Could you check a few things on this model? Use its own coordinates, in mm. A direction names the side the tool comes from. Give positions to 0.01 mm unless a question says otherwise; leave off trailing zeros. Loops run counter-clockwise (first coordinate to the right, second up) from the corner with the lowest first, then second, coordinate; pieces in that order, holes last. Notation, with made-up numbers: (44, -33.5) - (66, -33.5) arc R37 ccw to (66, 4.5) - close; hole circle Ø2 at (30, 29). An arc over 180 degrees is marked (long way). Write each question's results on one line, items separated by ' | '. Start each with the question number.
(1) Suppose I cut it at C-C (z = -11). Please give me the cut outline in (x, y).
(2) Suppose I cut it at A-A (z = -4.75). Please give me the cut outline in (x, y).
(3) If we mould it in two halves opening along Y, with no side actions, what happens to faces 6 (the face through (-6, 0, -6)), 7 (the face through (-7.3, 6, -10.3)), 8 (the face through (-1.25, 5, -6))? For each: released by +Y, released by -Y, zero draft, split by the parting line, or undercut.
(4) For pin 1 (1.2 mm diameter, centred on x = -6, y = 5, fed in from -Z); pin 2 (1.6 mm diameter, centred on x = -6, y = 5, fed in from +Z); pin 3 (0.8 mm diameter, centred on y = 5, z = -8.5, fed in from +X), each with a flat end and sliding along its axis, tell me the tip position at first contact or that it passes through.
(5) Suppose I cut it at B-B (x = -8.25). Please give me the cut outline in (y, z), and give its area (4 significant figures).
(6) On a 3-axis mill with a long thin cutter (end or side, diameter ignored), from which of +Z, -Z, +X, -X, +Y, -Y can I reach the whole of each face in a straight line? I mean faces 1 (the face through (0, 2, -6)), 2 (the face through (-6, 2, -12.55)), 3 (the face through (-6, 5, -11.25)), 4 (the face through (-6, 5, -1.25)), 5 (the face through (-11.25, 5, -6)). Say none if no direction works.
(7) Suppose I cut it at D-D (x = -0.75). Please give me the cut outline in (y, z), and give its area (3 significant figures).
(8) I need wall thicknesses on line 1 (Y direction, x = -8.75, z = -0.75); line 2 (Z direction, x = -1.75, y = 4.4). Which ranges of each line are inside material? Lowest first, please.
Autodesk Inventor part; units mm, degrees
ref_plane "YZ Plane" through (0, 0, 0) normal (1, 0, 0) x (0, 1, 0)
ref_plane "XZ Plane" through (0, 0, 0) normal (0, 1, 0) x (-1, 0, 0)
ref_plane "XY Plane" through (0, 0, 0) normal (0, 0, 1) x (1, 0, 0)
sketch "Sketch1" plane through (0, 0, 0) normal (0, 1, 0) x (-1, 0, 0)
  line L0 (0, 0) -> (12.5, 0)
  line L1 (12.5, 0) -> (12.5, -12.55)
  line L2 (12.5, -12.55) -> (0, -12.55)
  line L3 (0, -12.55) -> (0, 0)
  dimension "d0" = 12.5
  dimension "d1" = 12.55
extrude "Extrusion1" add sketch "Sketch1" along normal blind 4
sketch "Sketch2" plane through (0, 4, 0) normal (0, 1, 0) x (1, 0, 0)
  line L0 (-11.25, 1.25) -> (-1.25, 1.25)
  line L1 (-1.25, 1.25) -> (-1.25, 11.25)
  line L2 (-1.25, 11.25) -> (-11.25, 11.25)
  line L3 (-11.25, 11.25) -> (-11.25, 1.25)
  line L4 (-12.5, 0) -> (0, 0)
  line L5 (-12.5, 12.55) -> (-12.5, 0)
  dimension "d4" = 10
  dimension "d5" = 10
  dimension "d6" = 1.25
  dimension "d7" = 1.25
extrude "Extrusion2" add sketch "Sketch2" along normal blind 2
ref_plane "Work Plane1" through (-11.25, 4, -6.25) normal (0, 0, 1) x (1, 0, 0)
sketch "Sketch3" plane through (-11.25, 4, -6.25) normal (0, 0, 1) x (1, 0, 0)
  line L0 (10, 0) -> (0, 0)
  line L1 (10, 0) -> (10, 2)
  line L2 (0, 2) -> (10, 2)
  line L3 (0, 0) -> (0, 2)
  line L4 (5, 2) -> (5, 1.5)
  line L5 (5, 2) -> (9, 2)
  line L6 (5, 2) -> (1, 2)
  arc A0 (1, 2) -> (9, 2) centre (5, 17.75) ccw
  point P0 (11.25, -4)
  dimension "d10" = 0.5
  dimension "d11" = 4
  dimension "d12" = 4
revolve "Revolution1" cut sketch "Sketch3" angle 360 about axis through (-6.25, 6, -6.25) along (0, -1, 0) picked at (7.2273, 1.9076) contours A0 L4 L2
fillet "Fillet1" radius 0.5 4 edges at (-11.25, 6, -6.25) (-6.25, 6, -11.25) (-1.25, 6, -6.25) (-6.25, 6, -1.25)
properties part number "Top Button" material "PC/ABS Plastic"
Output values:
1) outline: (-12.5, 0) - (0, 0) - (0, 4) - (-1.25, 4) - (-1.25, 5.5) arc R0.5 ccw to (-1.5, 5.93) - (-11, 5.93) arc R0.5 ccw to (-11.25, 5.5) - (-11.25, 4) - (-12.5, 4) - close
2) outline: (-12.5, 0) - (0, 0) - (0, 4) - (-1.25, 4) - (-1.25, 5.5) arc R0.5 ccw to (-1.75, 6) - (-2.54, 6) arc R16.18 cw to (-9.96, 6) - (-10.75, 6) arc R0.5 ccw to (-11.25, 5.5) - (-11.25, 4) - (-12.5, 4) - close
3) face 6: released by -Y | face 7: released by +Y | face 8: zero draft
4) pin 1: z = -11.25 | pin 2: z = -1.25 | pin 3: x = -1.25
5) outline: (0, -12.55) - (4, -12.55) - (4, -11.25) - (5.5, -11.25) arc R0.5 ccw to (6, -10.75) - (6, -9.71) arc R16.13 cw to (6, -2.79) - (6, -1.75) arc R0.5 ccw to (5.5, -1.25) - (4, -1.25) - (4, 0) - (0, 0) - close | area: 68.35 mm2
6) face 1: +Z, -Z, +X, +Y, -Y | face 2: -Z, +X, -X, +Y, -Y | face 3: -Z, +X, -X, +Y | face 4: +Z, +X, -X, +Y | face 5: +Z, -Z, -X, +Y
7) outline: (0, -12.55) - (4, -12.55) - (4, 0) - (0, 0) - close | area: 50.2 mm2
8) line 1: 0 to 4 | line 2: -11.25 to -1.25
